```python
from build123d import *

# Parameters (mm, degrees)
SKETCH1_W                                            = 40
SKETCH1_H                                            = 60
BOSS_EXTRUDE1_DEPTH                                  = 10
CBORE_FOR_M3_HEX_SOCKET_THIN_HEAD_CAP_SC_D           = 3.4
CBORE_FOR_M3_HEX_SOCKET_THIN_HEAD_CAP_SC_CBORE_D     = 6.5
CBORE_FOR_M3_HEX_SOCKET_THIN_HEAD_CAP_SC_CBORE_DEPTH = 2.4
SKETCH4_R                                            = 15
CUT_EXTRUDE1_DEPTH                                   = 73.801098893


with BuildPart() as part:
    # Sketch1 → Boss-Extrude1 (new body)
    with BuildSketch(Plane(origin=(0, 0, 0), x_dir=(0, 0, -1), z_dir=(1, 0, 0))):
        with Locations((20, 30)):
            Rectangle(SKETCH1_W, SKETCH1_H)
    extrude(amount=BOSS_EXTRUDE1_DEPTH)

    # CBORE for M3 Hex Socket Thin Head Cap Screw1 (through all)
    with Locations(Plane(origin=(0, 0, 0), x_dir=(0, 0, -1), z_dir=(-1, 0, 0))):
        with Locations((5.857864376, -15.857864376), (5.857864376, -44.142135624), (34.142135624, -44.142135624), (34.142135624, -15.857864376)):
            CounterBoreHole(CBORE_FOR_M3_HEX_SOCKET_THIN_HEAD_CAP_SC_D / 2, CBORE_FOR_M3_HEX_SOCKET_THIN_HEAD_CAP_SC_CBORE_D / 2, CBORE_FOR_M3_HEX_SOCKET_THIN_HEAD_CAP_SC_CBORE_DEPTH)

    # Sketch4 → Cut-Extrude1 (cut, through all)
    with BuildSketch(Plane.ZY):
        with Locations((-20, 30)):
            Circle(SKETCH4_R)
    extrude(amount=-CUT_EXTRUDE1_DEPTH, mode=Mode.SUBTRACT)


solid = part.part
```
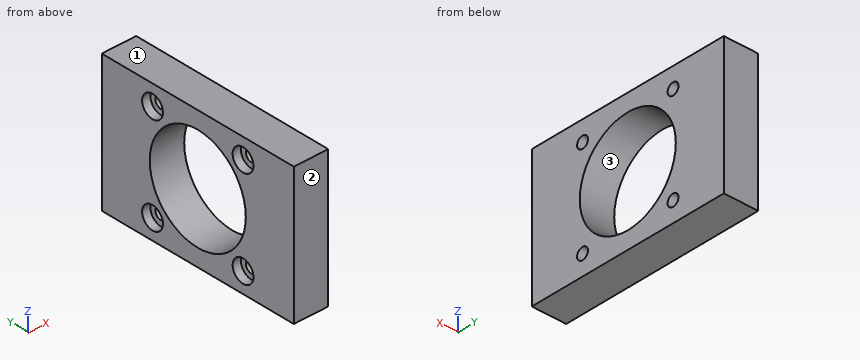
Build history of the part. All positions in model axes, mm. Face numbers are marked on the shaded views. Round coordinates to 2 decimals unless told otherwise and drop trailing zeros. Loops run counter-clockwise (first coordinate to the right, second up) from the corner with the lowest first, then second, coordinate; pieces in that order, holes last. Notation, with made-up numbers: M 83.5,32 L 130.5,32 A10 ccw 130.5,42 Z; hole C -12,51.5 d3. An arc over 180 degrees is marked long. Answer as CSV lines item,"result".
1. Flat gauge pins, fed straight in: P1, Ø1, axis at x = 7, y = 42, coming from the +Z side; P2, Ø2, axis at y = 17, z = -34, coming from the -X side; P3, Ø2.5, axis at y = 15.86, z = -5.86, coming from the -X side. Where does each tip first touch, or does it go through?
Resolved:
P1,"stops at z = 0"
P2,"stops at x = 2.4"
P3,"passes through"
2. Cut at A-A on z = -20. Write the cut outline in (x, y), then the cut area to 3 significant figures.
Resolved:
outline,"M 0,0 L 10,0 L 10,15 L 0,15 Z; M 0,45 L 10,45 L 10,60 L 0,60 Z"
area,"300 mm²"
3. Wall check: probe 1 along Y at (x, z) = (5, -4.5); probe 2 along Y at (x, z) = (6.5, -7); probe 3 along Z at (x, y) = (1.5, 17.5). Give the ranges that are in metal, low to high. Write a range as [from, to].
Resolved:
probe 1,"y = [0, 14.84], [16.88, 43.12], [45.16, 60]"
probe 2,"y = [0, 14.6], [17.12, 22.52], [37.48, 42.88], [45.4, 60]"
probe 3,"z = [-40, -36.95], [-31.34, -28.29], [-11.71, -8.66], [-3.05, 0]"
4. Cut at C-C on x = 1.75. Write the cut outline in (y, z).
Resolved:
outline,"M 0,-40 L 60,-40 L 60,0 L 0,0 Z; hole C 15.86,-34.14 d6.5; hole C 15.86,-5.86 d6.5; hole C 30,-20 d30; hole C 44.14,-34.14 d6.5; hole C 44.14,-5.86 d6.5"
5. Cut at D-D on x = 4.75. Write the cut outline in (y, z).
Resolved:
outline,"M 0,-40 L 60,-40 L 60,0 L 0,0 Z; hole C 15.86,-34.14 d3.4; hole C 15.86,-5.86 d3.4; hole C 30,-20 d30; hole C 44.14,-34.14 d3.4; hole C 44.14,-5.86 d3.4"
6. Cut at B-B on y = 30. Write the cut outline in (x, z), then the cut area to 3 significant figures.
Resolved:
outline,"M 0,-40 L 10,-40 L 10,-35 L 0,-35 Z; M 0,-5 L 10,-5 L 10,0 L 0,0 Z"
area,"100 mm²"
7. Two-plate mould, pull along Y, no slides. Class the marked faces 1, 2 and 3: released by +Y, released by -Y, zero draft, split by the parting line, or undercut.
Resolved:
face 1,"zero draft"
face 2,"released by -Y"
face 3,"undercut"
